Verification items for the finished model (mm, model axes). A direction names the side the tool comes from. Coordinates: 2 decimals unless noted, no trailing zeros. Order: outer loops, then holes, each group sorted by start corner. A loop starts at its lowest first (then second) coordinate and runs counter-clockwise, first axis right, second up. Notation, with made-up numbers: M 18.5,14 L 44.5,14 A10 cw 44.5,24 Z; hole C -30.75,-13.75 d4. An arc over 180 degrees is marked long. Use one line per item in the form item = value. Start each with the question number.
```python
from build123d import *

# Parameters (mm, degrees)
F0_R     = 29.972
F0_W     = 29.6613248065
F0_H     = 27.7720661834
F1_DEPTH = 59.944
F2_DEPTH = 25.4


with BuildPart() as f1:
    # F0 (on Top) → F1 (new body)
    with BuildSketch(Plane.XY):
        Circle(F0_R)
        with Locations((0.330620911, -0.7084705867)):
            Rectangle(F0_W, F0_H, mode=Mode.SUBTRACT)
    extrude(amount=F1_DEPTH)

    # F2 (add): a face of the model
    f2_faces = [f1.faces().sort_by_distance(p)[0] for p in [
        (-14.5000414923, -0.7084705867, 29.972),
    ]]
    extrude(f2_faces, amount=F2_DEPTH)


solid = f1.part
```
1. Material ranges on line 1 along X through (y, z) = (1, 45.5); line 2 along X through (y, z) = (-11, 54); line 3 along Y through (x, z) = (12, 2), recorded low to high.
2. Cross-section at B-B on z = 30.5. Enter the section's corners in (x, y).
3. Release check for a two-part mould opening along Y. For faces 1 (the flat face through (0, 0, 59.944)), 2 (the flat face through (15.161, -1, 30)), 3 (the cylindrical face through (-3.902, 29.717, 29.552)) record: pulls with the +Y half, pulls with the -Y half, needs draft (parallel to the pull), parting line crosses it, or undercut.
4. Cross-section at D-D on y = 21. Enter the section's corners in (x, z).
5. Depth check by flat-ended pin: P1, Ø1.5, axis at y = 13, z = 50.5, coming from the +X side; P2, Ø8, axis at x = -5, z = 46, coming from the +Y side; P3, Ø2, axis at x = 12.5, z = 21, coming from the +Y side. Enter the tip coordinate at first touch or a pass-through.
6. Cross-section at A-A on y = 0. Enter the section's corners in (x, z), and give its area (3 significant figures).
7. Tool access check on faces 4 (the flat face through (0, 0, 0)), 5 (the flat face through (13, -14.595, 30)). Record the directions out of +Z, -Z, +X, -X, +Y, -Y that give a thin tool (end or side, any length) a straight path to the whole face; none if there is none.
8. Cross-section at C-C on x = 25.5. Enter the section's corners in (y, z).
Final values:
q1.line_1 = -29.96 to 10.9, 15.16 to 29.96
q1.line_2 = -27.88 to 10.9, 15.16 to 27.88
q1.line_3 = -27.46 to -14.59, 13.18 to 27.46
q2.outline = C 0,0 d59.94; hole M 10.9,-14.59 L 15.16,-14.59 L 15.16,13.18 L 10.9,13.18 Z
q3.face_1 = needs draft
q3.face_2 = undercut
q3.face_3 = parting line crosses it
q4.outline = M -21.39,0 L 21.39,0 L 21.39,59.94 L -21.39,59.94 Z
q5.P1 = 27.35
q5.P2 = 29.96
q5.P3 = 27.68
q6.outline = M -29.97,0 L 10.9,0 L 10.9,59.94 L -29.97,59.94 Z; M 15.16,0 L 29.97,0 L 29.97,59.94 L 15.16,59.94 Z
q6.area = 3,340 mm2
q7.face_4 = -Z, +X, -X, +Y, -Y
q7.face_5 = +Z, -Z
q8.outline = M -15.75,0 L 15.75,0 L 15.75,59.94 L -15.75,59.94 Z
